The model under review builds one solid part; all positions refer to its coordinate system, in mm. Face numbers are marked on the shaded views. Coordinates: 2 decimals unless noted, no trailing zeros. Loops run counter-clockwise (first coordinate to the right, second up) from the corner with the lowest first, then second, coordinate; pieces in that order, holes last. Notation, with made-up numbers: (62, -6) - (104, -6) arc R26 cw to (104, 28) - close; hole circle Ø2 at (13.5, 12.25). An arc over 180 degrees is marked (long way). One line per item, written item: value. Start each with the question number.
1. Mouldability with a two-part tool opening along X and no side actions: class the marked faces 1, 2, 3 and 4 as +X half, -X half, draft (parallel to the pull), parting line (faces both ways), or undercut.
2. We need section B-B, the plane y = -13.5. Give the boundary of the cut face in (x, z) (3 decimals).
3. We need section A-A, the plane x = -30. Give the boundary of the cut face in (y, z) (3 decimals), then the cut area to 3 significant figures.
4. Insertion check: P1, Ø4, axis at x = 30, y = -13.5, coming from the -Z side. The pin has a flat end and moves straight along its axis. Give the tip position at first contact, or say it passes through.
5. To check wall thickness, follow line 1 (Y direction, x = 30, z = 13.25) (3 decimals); line 2 (Y direction, x = 30, z = -7.75); line 3 (Z direction, x = -29, y = -7.25). State the ranges of each line that lie inside material, in increasing order.
6. We need section D-D, the plane z = 12.75. Give the boundary of the cut face in (x, y) (3 decimals), then the cut area to 3 significant figures.
7. We need section C-C, the plane x = 30. Give the boundary of the cut face in (y, z) (3 decimals), then the cut area to 3 significant figures.
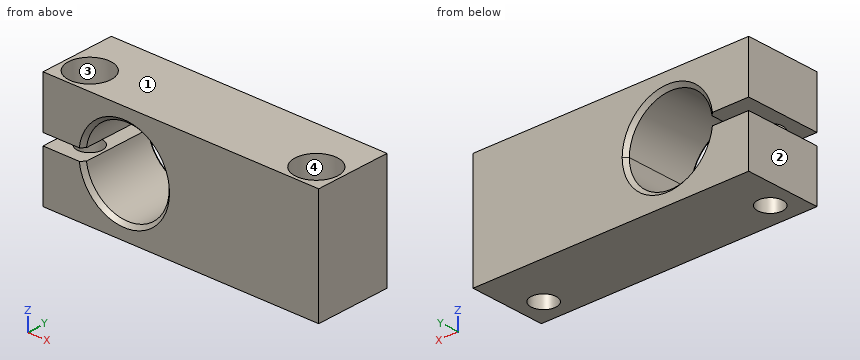
from build123d import *

# Parameters (mm, degrees)
F1_DEPTH       = 20
F3_D           = 6.6
F3_CBORE_D     = 11.25
F3_CBORE_DEPTH = 6
F4_SIZE        = 1


with BuildPart() as f1:
    # F0 (on Front) → F1 (new body)
    with BuildSketch(Plane.XZ):
        with BuildLine():
            Line((36.5, 15), (-36.5, 15))
            Line((-36.5, 15), (-36.5, 1.5))
            Line((-36.5, 1.5), (-25.8972473589, 1.5))
            ThreePointArc((-25.8972473589, 1.5), (-14.2482423753, 10.9742817748), (-4, 0))
            ThreePointArc((-4, 0), (-14.2482423753, -10.9742817748), (-25.8972473589, -1.5))
            Line((-25.8972473589, -1.5), (-36.5, -1.5))
            Line((-36.5, -1.5), (-36.5, -15))
            Line((-36.5, -15), (36.5, -15))
            Line((36.5, -15), (36.5, 15))
        make_face()
    extrude(amount=F1_DEPTH)

    # F3 (through all)
    with Locations(Plane.XY.offset(15)):
        with Locations((-30, -13.5), (30, -13.5)):
            CounterBoreHole(F3_D / 2, F3_CBORE_D / 2, F3_CBORE_DEPTH)

    # F4
    f4_edges = [f1.edges().sort_by_distance(p)[0] for p in [
        (-4, -20, 0),
        (-4, 0, 0),
    ]]
    chamfer(f4_edges, length=F4_SIZE)


solid = f1.part
Findings below:
1. face 1: draft
1. face 2: -X half
1. face 3: undercut
1. face 4: undercut
2. outline: (-36.5, -15) - (-33.3, -15) - (-33.3, -1.5) - (-36.5, -1.5) - close; (-36.5, 1.5) - (-33.3, 1.5) - (-33.3, 9) - (-35.625, 9) - (-35.625, 15) - (-36.5, 15) - close; (-26.7, -15) - (26.7, -15) - (26.7, 9) - (24.375, 9) - (24.375, 15) - (-24.375, 15) - (-24.375, 9) - (-26.7, 9) - (-26.7, 1.5) - (-25.897, 1.5) arc R11 cw (long way) to (-25.897, -1.5) - (-26.7, -1.5) - close; (33.3, -15) - (36.5, -15) - (36.5, 15) - (35.625, 15) - (35.625, 9) - (33.3, 9) - close
3. outline: (-20, -15) - (-16.8, -15) - (-16.8, -1.5) - (-20, -1.5) - close; (-20, 1.5) - (-16.8, 1.5) - (-16.8, 9) - (-19.125, 9) - (-19.125, 15) - (-20, 15) - close; (-10.2, -15) - (0, -15) - (0, -1.5) - (-10.2, -1.5) - close; (-10.2, 1.5) - (0, 1.5) - (0, 15) - (-7.875, 15) - (-7.875, 9) - (-10.2, 9) - close
3. area: 334 mm2
4. P1: through
5. line 1: -20 to -19.125, -7.875 to 0
5. line 2: -20 to -16.8, -10.2 to 0
5. line 3: -15 to -1.5, 1.5 to 15
6. outline: (-36.5, -20) - (36.5, -20) - (36.5, 0) - (-36.5, 0) - close; hole circle Ø11.25 at (-30, -13.5); hole circle Ø11.25 at (30, -13.5)
6. area: 1,260 mm2
7. outline: (-20, -15) - (-16.8, -15) - (-16.8, 9) - (-19.125, 9) - (-19.125, 15) - (-20, 15) - close; (-10.2, -15) - (0, -15) - (0, 15) - (-7.875, 15) - (-7.875, 9) - (-10.2, 9) - close
7. area: 374 mm2
